Can you work these out from the model? Positions are in its coordinate system, mm. A direction names the side the tool comes from. Round coordinates to 2 decimals unless told otherwise and drop trailing zeros. Order: outer loops, then holes, each group sorted by start corner. A loop starts at its lowest first (then second) coordinate and runs counter-clockwise, first axis right, second up. Notation, with made-up numbers: M 34.5,81 L 58.5,81 A21 cw 58.5,88 Z; hole C -33.5,50.5 d3. An arc over 180 degrees is marked long. Answer as a JSON object with one key per item and string values. Group by question number.
from build123d import *

# Parameters (mm, degrees)
F0_W      = 100
F0_H      = 35
F1_DEPTH  = 50
F3_DEPTH  = 35.001
F4_W      = 90
F4_H      = 25
F5_DEPTH  = 30
F6_R      = 1.575
F7_DEPTH  = 50.001
F9_DEPTH  = 18
F10_W     = 20
F10_H     = 5
F11_DEPTH = 25
F12_W     = 25
F12_H     = 25
F13_DEPTH = 100.001
F14_W     = 3
F14_H     = 10
F14_W_2   = 10
F14_H_2   = 3
F15_DEPTH = 5
F16_R     = 1.575
F17_DEPTH = 5.001
F18_W     = 31
F18_H     = 3
F19_DEPTH = 3


with BuildPart() as f1:
    # F0 (on Top) → F1 (new body)
    with BuildSketch(Plane.XY):
        Rectangle(F0_W, F0_H)
    extrude(amount=F1_DEPTH)

    # F2 (on face) → F3 (cut, through all)
    with BuildSketch(Plane.XZ.offset(17.5)):
        with BuildLine():
            Line((0, 9), (-45, 9))
            ThreePointArc((-45, 9), (-47, 7), (-45, 5))
            Line((-45, 5), (0, 5))
            Line((0, 5), (45, 5))
            ThreePointArc((45, 5), (47, 7), (45, 9))
            Line((45, 9), (0, 9))
        make_face()
        with BuildLine():
            Line((0, 26), (45, 26))
            ThreePointArc((45, 26), (47, 28), (45, 30))
            Line((45, 30), (0, 30))
            Line((0, 30), (-45, 30))
            ThreePointArc((-45, 30), (-47, 28), (-45, 26))
            Line((-45, 26), (0, 26))
        make_face()
    extrude(amount=-F3_DEPTH, mode=Mode.SUBTRACT)

    # F4 (on face) → F5 (cut)
    with BuildSketch(Plane(origin=(0, 0, 0), x_dir=(1, 0, 0), z_dir=(0, 0, -1))):
        Rectangle(F4_W, F4_H)
    extrude(amount=-F5_DEPTH, mode=Mode.SUBTRACT)

    # F6 (on face) → F7 (cut, through all)
    with BuildSketch(Plane.XY.offset(50)):
        with Locations((-42.5, 5)):
            Circle(F6_R)
        with Locations((-42.5, -5)):
            Circle(F6_R)
        with Locations((-37.5, 5)):
            Circle(F6_R)
        with Locations((-37.5, -5)):
            Circle(F6_R)
        with Locations((-32.5, 5)):
            Circle(F6_R)
        with Locations((-32.5, -5)):
            Circle(F6_R)
        with Locations((-27.5, 5)):
            Circle(F6_R)
        with Locations((-27.5, -5)):
            Circle(F6_R)
        with Locations((-22.5, 5)):
            Circle(F6_R)
        with Locations((-22.5, -5)):
            Circle(F6_R)
        with Locations((-17.5, 5)):
            Circle(F6_R)
        with Locations((-17.5, -5)):
            Circle(F6_R)
        with Locations((-12.5, 5)):
            Circle(F6_R)
        with Locations((-12.5, -5)):
            Circle(F6_R)
        with Locations((-7.5, 5)):
            Circle(F6_R)
        with Locations((-7.5, -5)):
            Circle(F6_R)
        with Locations((-2.5, 5)):
            Circle(F6_R)
        with Locations((-2.5, -5)):
            Circle(F6_R)
        with Locations((2.5, 5)):
            Circle(F6_R)
        with Locations((2.5, -5)):
            Circle(F6_R)
        with Locations((7.5, 5)):
            Circle(F6_R)
        with Locations((7.5, -5)):
            Circle(F6_R)
        with Locations((12.5, 5)):
            Circle(F6_R)
        with Locations((12.5, -5)):
            Circle(F6_R)
        with Locations((17.5, 5)):
            Circle(F6_R)
        with Locations((17.5, -5)):
            Circle(F6_R)
        with Locations((22.5, 5)):
            Circle(F6_R)
        with Locations((22.5, -5)):
            Circle(F6_R)
        with Locations((27.5, 5)):
            Circle(F6_R)
        with Locations((27.5, -5)):
            Circle(F6_R)
        with Locations((32.5, 5)):
            Circle(F6_R)
        with Locations((32.5, -5)):
            Circle(F6_R)
        with Locations((37.5, 5)):
            Circle(F6_R)
        with Locations((37.5, -5)):
            Circle(F6_R)
        with Locations((42.5, 5)):
            Circle(F6_R)
        with Locations((42.5, -5)):
            Circle(F6_R)
    extrude(amount=-F7_DEPTH, mode=Mode.SUBTRACT)

    # F8 (on face) → F9 (cut)
    with BuildSketch(Plane.XY.offset(50)):
        with BuildLine():
            Line((45, 9), (-45, 9))
            ThreePointArc((-45, 9), (-49, 5), (-45, 1))
            Line((-45, 1), (45, 1))
            ThreePointArc((45, 1), (49, 5), (45, 9))
        make_face()
        with BuildLine():
            ThreePointArc((-45, -1), (-49, -5), (-45, -9))
            Line((-45, -9), (45, -9))
            ThreePointArc((45, -9), (49, -5), (45, -1))
            Line((45, -1), (-45, -1))
        make_face()
    extrude(amount=-F9_DEPTH, mode=Mode.SUBTRACT)

    # F10 (on face) → F11 (join)
    with BuildSketch(Plane.XZ.offset(-12.5)):
        with Locations((-25, 2.5)):
            Rectangle(F10_W, F10_H)
        with Locations((25, 2.5)):
            Rectangle(F10_W, F10_H)
    extrude(amount=F11_DEPTH)

    # F12 (on face) → F13 (cut, through all)
    with BuildSketch(Plane.YZ.offset(50)):
        with Locations((0, 17.5)):
            Rectangle(F12_W, F12_H)
    extrude(amount=-F13_DEPTH, mode=Mode.SUBTRACT)

    # F14 (on face) → F15 (join)
    with BuildSketch(Plane.XZ.offset(17.5)):
        with Locations((-14, 35)):
            Rectangle(F14_W, F14_H)
        with Locations((14, 35)):
            Rectangle(F14_W, F14_H)
        with Locations((0, 48.5)):
            Rectangle(F14_W_2, F14_H_2)
        with Locations((0, 20.5)):
            Rectangle(F14_W_2, F14_H_2)
    extrude(amount=F15_DEPTH)

    # F16 (on face) → F17 (cut, through all)
    with BuildSketch(Plane.XY.offset(5)):
        with Locations((-32.5, 5)):
            Circle(F16_R)
        with Locations((-27.5, 5)):
            Circle(F16_R)
        with Locations((-22.5, 5)):
            Circle(F16_R)
        with Locations((-17.5, 5)):
            Circle(F16_R)
        with Locations((-32.5, -5)):
            Circle(F16_R)
        with Locations((-22.5, -5)):
            Circle(F16_R)
        with Locations((-27.5, -5)):
            Circle(F16_R)
        with Locations((-17.5, -5)):
            Circle(F16_R)
        with Locations((17.5, 5)):
            Circle(F16_R)
        with Locations((17.5, -5)):
            Circle(F16_R)
        with Locations((22.5, 5)):
            Circle(F16_R)
        with Locations((22.5, -5)):
            Circle(F16_R)
        with Locations((27.5, 5)):
            Circle(F16_R)
        with Locations((27.5, -5)):
            Circle(F16_R)
        with Locations((32.5, 5)):
            Circle(F16_R)
        with Locations((32.5, -5)):
            Circle(F16_R)
    extrude(amount=-F17_DEPTH, mode=Mode.SUBTRACT)

    # F18 (on face) → F19 (join)
    with BuildSketch(Plane.XZ.offset(22.5)):
        with Locations((0, 31.5)):
            Rectangle(F18_W, F18_H)
    extrude(amount=F19_DEPTH)


solid = f1.part
Item 1: Suppose I cut it at B-B, the plane y = 10.5. Write out the boundary of the cut face in (x, z).
Item 2: Suppose I cut it at A-A, the plane z = 18. Write out the boundary of the cut face in (x, y).
Item 3: On a 3-axis mill with a long thin cutter (end or side, diameter ignored), from which of +Z, -Z, +X, -X, +Y, -Y can I reach the whole of each face in a straight line? I mean faces 4 (the face through (-49, 5, 41)), 5 (the face through (1, 15, 9)), 6 (the face through (35, 0, 2)). Say none if no direction works.
Item 4: I need wall thicknesses on line 1 (X direction, y = 11.5, z = 2); line 2 (Y direction, x = 17.5, z = 31.35) (3 decimals); line 3 (Y direction, x = -16, z = 47.5). Which ranges of each line are inside material? Lowest first, please.
Item 5: Suppose I cut it at C-C, the plane z = 7. Write out the boundary of the cut face in (x, y).
Item 6: I'm going to push flat-ended pins straight in: pin 1 Ø3 at (x, y) = (7.5, -5) entering from -Z; pin 2 Ø8 at (x, y) = (2.5, -3) entering from -Z; pin 3 Ø5 at (x, y) = (-42.5, 5) entering from +Z; pin 4 Ø1.5 at (x, z) = (-19, 24) entering from -Y. Where does each tip first touch, or does it pass through?
Item 7: Suppose I cut it at D-D, the plane z = 41.5. Write out the boundary of the cut face in (x, y).
Item 8: If we mould it in two halves opening along Z, with no side actions, what happens to faces 1 (the face through (47, -15, 7)), 2 (the face through (-23, 0, 0)), 3 (the face through (-2.71, -3.44, 31.01))? For each: +Z half, -Z half, draft (parallel to the pull), parting line (faces both ways), or undercut.
Computed:
{
 "1": {"outline": "M -50,0 L -45,0 L -45,5 L -50,5 Z; M -50,30 L 50,30 L 50,50 L -50,50 Z; M -35,0 L -15,0 L -15,5 L -35,5 Z; M 15,0 L 35,0 L 35,5 L 15,5 Z; M 45,0 L 50,0 L 50,5 L 45,5 Z"},
 "2": {"outline": "M -50,-17.5 L 50,-17.5 L 50,-12.5 L -50,-12.5 Z; M -50,12.5 L 50,12.5 L 50,17.5 L -50,17.5 Z"},
 "3": {"face 4": "+Z", "face 5": "+Y, -Y", "face 6": "-Z"},
 "4": {"line 1": "x = -50 to -45, -35 to -15, 15 to 35, 45 to 50", "line 2": "y = -17.5 to -6.575, -3.425 to 3.425, 6.575 to 17.5", "line 3": "y = -17.5 to -9, -1 to 1, 9 to 17.5"},
 "5": {"outline": "M -50,-17.5 L -47,-17.5 L -47,-12.5 L -50,-12.5 Z; M -50,12.5 L -47,12.5 L -47,17.5 L -50,17.5 Z; M 47,-17.5 L 50,-17.5 L 50,-12.5 L 47,-12.5 Z; M 47,12.5 L 50,12.5 L 50,17.5 L 47,17.5 Z"},
 "6": {"pin 1": "passes through", "pin 2": "stops at z = 30", "pin 3": "stops at z = 32", "pin 4": "stops at y = -17.5"},
 "7": {"outline": "M -50,-17.5 L 50,-17.5 L 50,17.5 L -50,17.5 Z; hole M -45,-9 L 45,-9 A4 ccw 45,-1 L -45,-1 A4 ccw Z; hole M -45,1 L 45,1 A4 ccw 45,9 L -45,9 A4 ccw Z"},
 "8": {"face 1": "undercut", "face 2": "-Z half", "face 3": "draft"}
}
